```python
from build123d import *

# Parameters (mm, degrees)
SKETCH_1_R           = 6
EXTRUDE_1_DEPTH      = 70
EXTRUDE_1_DEPTH_BACK = 10
SKETCH_3_W           = 1
SKETCH_3_H           = 0.5


with BuildPart() as part:
    # 草图1 → 凸台-拉伸1 (new body, two sides)
    with BuildSketch(Plane.XY) as extrude_1_sk:
        Circle(SKETCH_1_R)
    extrude(amount=EXTRUDE_1_DEPTH)
    extrude(extrude_1_sk.sketch, amount=-EXTRUDE_1_DEPTH_BACK)

    # 草图3 → 切除-旋转1 (revolve, cut)
    with BuildSketch(Plane(origin=(0, 0, 0), x_dir=(0, 0, -1), z_dir=(1, 0, 0))):
        with Locations((-65.5, 5.75)):
            Rectangle(SKETCH_3_W, SKETCH_3_H)
    revolve(axis=Axis((0, 0, 70), (0, 0, -1)), mode=Mode.SUBTRACT)


solid = part.part
```
CAD build for the part. Positions are in the model's coordinates, mm. A direction names the side the tool comes from. Coordinates: 2 decimals unless noted, no trailing zeros. Write each loop counter-clockwise with the first axis right and the second up, starting at its lowest first coordinate (ties: lowest second). Pieces come first, ordered by that corner, then holes. Notation, with made-up numbers: (18, -14.75) -> (43, -14.75) arc R27 ccw to (43, 12.25) -> close; hole circle Ø7 at (-33, 10). An arc over 180 degrees is marked (long way). Return JSON: item names as keys, results as strings. Group by question number.
Q1. Cut at A-A, the plane y = 2.75. Give the cut face in (x, z).
Q2. Cut at B-B, the plane x = -3.75. Give the cut face in (y, z), then the cut area to 3 significant figures.
Q3. Cut at C-C, the plane z = 28. Give the cut face in (x, y), then the cut area to 3 significant figures.
Q4. Which spindle directions (+Z, -Z, +X, -X, +Y, -Y) get a long thin tool onto all of the face, cutting with end or side? Do faces 1 (the face through (-5.37, -1.19, 65.49)), 2 (the face through (5.54, -2.3, 28.02)). Say none if no direction does.
Q5. Pull direction Z, two halves, no side cores. Call faces 3 (the face through (-5, -3, 66)), 4 (the face through (0, 0, -10)), 5 (the face through (-5, -3, 65)), 6 (the face through (5.54, -2.3, 68.03)): released by +Z, released by -Z, zero draft, split by the parting line, or undercut.
Q6. Drill centre lines: line 1 (Z direction, x = -3.25, y = -4.75); line 2 (X direction, y = -0.25, z = 51); line 3 (Y direction, x = 3.25, z = 32.5). Where is each one in solid material? Low to high.
Q7. Flat gauge pins, fed straight in: pin 1 (1.5 mm diameter, centred on y = 3.5, z = 10.5, fed in from -X); pin 2 (1.5 mm diameter, centred on x = 2.5, z = 52.5, fed in from +Y). Where does each tip first touch, or does it go through?
Returned:
{
 "1": {"outline": "(-5.33, -10) -> (5.33, -10) -> (5.33, 65) -> (4.76, 65) -> (4.76, 66) -> (5.33, 66) -> (5.33, 70) -> (-5.33, 70) -> (-5.33, 66) -> (-4.76, 66) -> (-4.76, 65) -> (-5.33, 65) -> close"},
 "2": {"outline": "(-4.68, -10) -> (4.68, -10) -> (4.68, 65) -> (4.02, 65) -> (4.02, 66) -> (4.68, 66) -> (4.68, 70) -> (-4.68, 70) -> (-4.68, 66) -> (-4.02, 66) -> (-4.02, 65) -> (-4.68, 65) -> close", "area": "748 mm2"},
 "3": {"outline": "circle Ø12 at (0, 0)", "area": "113 mm2"},
 "4": {"face 1": "none", "face 2": "+Z, -Z"},
 "5": {"face 3": "undercut", "face 4": "released by -Z", "face 5": "undercut", "face 6": "zero draft"},
 "6": {"line 1": "z = -10 to 65, 66 to 70", "line 2": "x = -5.99 to 5.99", "line 3": "y = -5.04 to 5.04"},
 "7": {"pin 1": "stops at x = -5.33", "pin 2": "stops at y = 5.74"}
}
